Check sheet for the modelled part. Datum: model origin and axes. Units: mm. Face numbers are marked on the shaded views. Coordinates: 2 decimals unless noted, no trailing zeros. Loops run counter-clockwise (first coordinate to the right, second up) from the corner with the lowest first, then second, coordinate; pieces in that order, holes last.
from build123d import *

# Parameters (mm, degrees)
UPPER_START               = 58
SKETCH1_W                 = 66
SKETCH1_H                 = 92.5
SKETCH1_R                 = 18
SKETCH1_R_2               = 2.3
UPPER_BEARING_PLATE_DEPTH = 7


with BuildPart() as part:
    # Sketch1 → Upper bearing plate (new body)
    with BuildSketch(Plane.XY.offset(UPPER_START)):
        Rectangle(SKETCH1_W, SKETCH1_H)
        Circle(SKETCH1_R, mode=Mode.SUBTRACT)
        with Locations((-28, -40.5)):
            Circle(SKETCH1_R_2, mode=Mode.SUBTRACT)
        with Locations((-28, 40.5)):
            Circle(SKETCH1_R_2, mode=Mode.SUBTRACT)
        with Locations((28, -40.5)):
            Circle(SKETCH1_R_2, mode=Mode.SUBTRACT)
        with Locations((28, 40.5)):
            Circle(SKETCH1_R_2, mode=Mode.SUBTRACT)
    extrude(amount=UPPER_BEARING_PLATE_DEPTH)


solid = part.part
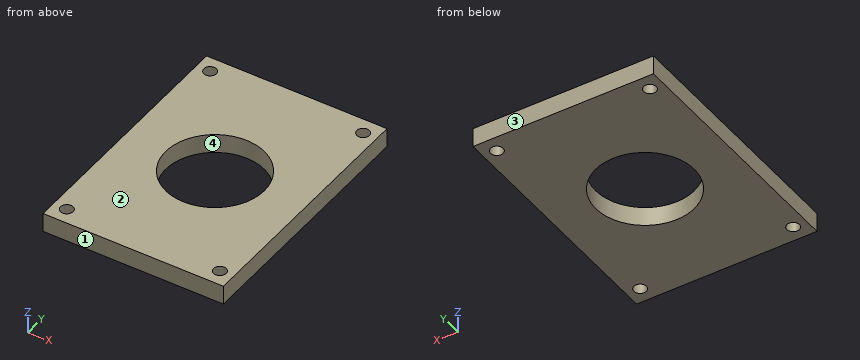
(1) Scan lines: line 1 along Y through (x, z) = (-28, 63.5); line 2 along X through (y, z) = (41, 63) (3 decimals); line 3 along Y through (x, z) = (0, 63). Record each from-to range of solid material in increasing order.
(2) Section check C-C, the plane x = 0. Enter the section's corners in (y, z).
(3) Section check B-B, the plane y = 40.5. Enter the section's corners in (x, z).
(4) Section check D-D, the plane z = 62. Enter the section's corners in (x, y).
(5) Draft check along Y on the marked faces 1, 2, 3 and 4. Enter one of: pulls with the +Y half, pulls with the -Y half, needs draft (parallel to the pull), parting line crosses it, or undercut.
(6) Section check A-A, the plane x = 28. Enter the section's corners in (y, z), plus the area to 3 significant figures.
(7) Gauge pin test, flat end, axial feed: P1, Ø4, axis at x = -28, y = -40.5, coming from the +Z side. Record the tip position at first contact, or that the pin passes through.
Determined:
1. line 1: y = -46.25 to -42.8, -38.2 to 38.2, 42.8 to 46.25
1. line 2: x = -33 to -30.245, -25.755 to 25.755, 30.245 to 33
1. line 3: y = -46.25 to -18, 18 to 46.25
2. outline: (-46.25, 58) - (-18, 58) - (-18, 65) - (-46.25, 65) - close; (18, 58) - (46.25, 58) - (46.25, 65) - (18, 65) - close
3. outline: (-33, 58) - (-30.3, 58) - (-30.3, 65) - (-33, 65) - close; (-25.7, 58) - (25.7, 58) - (25.7, 65) - (-25.7, 65) - close; (30.3, 58) - (33, 58) - (33, 65) - (30.3, 65) - close
4. outline: (-33, -46.25) - (33, -46.25) - (33, 46.25) - (-33, 46.25) - close; hole circle Ø4.6 at (-28, -40.5); hole circle Ø4.6 at (-28, 40.5); hole circle Ø36 at (0, 0); hole circle Ø4.6 at (28, -40.5); hole circle Ø4.6 at (28, 40.5)
5. face 1: pulls with the -Y half
5. face 2: needs draft
5. face 3: pulls with the +Y half
5. face 4: undercut
6. outline: (-46.25, 58) - (-42.8, 58) - (-42.8, 65) - (-46.25, 65) - close; (-38.2, 58) - (38.2, 58) - (38.2, 65) - (-38.2, 65) - close; (42.8, 58) - (46.25, 58) - (46.25, 65) - (42.8, 65) - close
6. area: 583 mm2
7. P1: passes through
